Here's how the part is built. I have some questions about the finished solid (model axes, mm). A direction names the side the tool comes from. Coordinates: 2 decimals unless noted, no trailing zeros. Write each loop counter-clockwise with the first axis right and the second up, starting at its lowest first coordinate (ties: lowest second). Pieces come first, ordered by that corner, then holes.
Item 1: For faces 4 (the face through (18.255, 1.479, 74.828)), 5 (the face through (-1, 18, 98)), which set-ups out of +Z, -Z, +X, -X, +Y, -Y let a thin tool reach every point of the face, with its end or its side?
Item 2: If we mould it in two halves opening along Y, with no side actions, what happens to faces 1 (the face through (-48.4, 33, -0.5)), 2 (the face through (-1.08, 1.48, 77.46)), 3 (the face through (-1.92, 12.12, -99.01))? For each: pulls with the +Y half, pulls with the -Y half, needs draft (parallel to the pull), parting line crosses it, or undercut.
Item 3: I want a section at C-C (z = 22). Please give me the cut outline in (x, y).
Item 4: I want a section at A-A (z = -80). Please give me the cut outline in (x, y).
Item 5: Please list where these lines run through material, in increasing order: line 1 (Z direction, x = -43, y = 12.5); line 2 (X direction, y = 1, z = -26); line 3 (X direction, y = 24, z = -77).
Item 6: I want a section at B-B (x = -21). Please give me the cut outline in (y, z).
Item 7: I'm going to push flat-ended pins straight in: P1, Ø1.5, axis at x = 7, z = 65.5, coming from the -Y side; P2, Ø2, axis at x = -23, z = 25.5, coming from the +Y side. Where does each tip first touch, or does it pass through?
Item 8: I want a section at D-D (y = 25). Please give me the cut outline in (x, z), and give its area (3 significant figures).
Autodesk Inventor part; units mm, degrees
ref_plane "YZ Plane" through (0, 0, 0) normal (1, 0, 0) x (0, 1, 0)
ref_plane "XZ Plane" through (0, 0, 0) normal (0, 1, 0) x (-1, 0, 0)
ref_plane "XY Plane" through (0, 0, 0) normal (0, 0, 1) x (1, 0, 0)
sketch "스케치1" plane through (0, 0, 0) normal (0, 1, 0) x (-1, 0, 0)
  line L0 (50, 100) -> (-50, 100)
  line L1 (-50, 100) -> (-50, -100)
  line L2 (-50, -100) -> (50, -100)
  line L3 (50, -100) -> (50, 100)
  point P0 (0, 0)
  dimension "d0" = 100
  dimension "d1" = 200
extrude "돌출1" add sketch "스케치1" along normal blind 3
sketch "스케치2" plane through (0, 0, 0) normal (0, -1, 0) x (1, 0, 0)
  circle A0 centre (25, 80) radius 8.5
  circle A1 centre (35, 63) radius 1.6
  circle A2 centre (15, 63) radius 1.6
  circle A3 centre (-5, 85) radius 8.5
  circle A4 centre (4.25, 63) radius 1.6
  circle A5 centre (-14.25, 63) radius 1.6
  circle A6 centre (-35, 85) radius 8.5
  circle A7 centre (-26.25, 63) radius 1.6
  circle A8 centre (-43.75, 63) radius 1.6
  line L0 (-50, 100) -> (50, 100)
  line L1 (-50, -100) -> (-50, 100)
  line L2 (45, 30) -> (5, 30)
  line L3 (5, 30) -> (5, 10)
  line L4 (5, 10) -> (45, 10)
  line L5 (45, 10) -> (45, 30)
  circle A9 centre (2.5, 28.5) radius 1.6
  circle A10 centre (43.5, -4.5) radius 1.6
  circle A11 centre (35, 20) radius 9.6 construction
  line L6 (7, 95) -> (-17, 95) construction
  line L7 (-17, 95) -> (-17, 61) construction
  line L8 (-17, 61) -> (7, 61) construction
  line L9 (7, 61) -> (7, 95) construction
  line L10 (38.25, 96) -> (11.75, 96) construction
  line L11 (11.75, 96) -> (11.75, 60) construction
  line L12 (11.75, 60) -> (38.25, 60) construction
  line L13 (38.25, 60) -> (38.25, 96) construction
  line L14 (-23.5, 95) -> (-46.5, 95) construction
  line L15 (-46.5, 95) -> (-46.5, 61) construction
  line L16 (-46.5, 61) -> (-23.5, 61) construction
  line L17 (-23.5, 61) -> (-23.5, 95) construction
  line L18 (46.5, -24) -> (3.5, -24) construction
  line L19 (3.5, -24) -> (3.5, -96) construction
  line L20 (3.5, -96) -> (46.5, -96) construction
  line L21 (46.5, -96) -> (46.5, -24) construction
  line L22 (46.5, -24) -> (3.5, -96) construction
  line L23 (3.5, -24) -> (46.5, -96) construction
  line L24 (44.5, -29) -> (5.5, -29)
  line L25 (5.5, -29) -> (5.5, -91)
  line L26 (5.5, -91) -> (44.5, -91)
  line L27 (44.5, -91) -> (44.5, -29)
  line L28 (44.5, -29) -> (5.5, -91) construction
  line L29 (5.5, -29) -> (44.5, -91) construction
  circle A12 centre (44.4, -93.5) radius 1.5
  circle A13 centre (5.6, -93.5) radius 1.5
  circle A14 centre (5.6, -26.5) radius 1.5
  circle A15 centre (44.4, -26.5) radius 1.5
  line L30 (-29, 29.5) -> (-48, 29.5) construction
  line L31 (-48, 29.5) -> (-48, 14.5) construction
  line L32 (-48, 14.5) -> (-29, 14.5) construction
  line L33 (-29, 14.5) -> (-29, 29.5) construction
  circle A16 centre (-40, 22) radius 3
  circle A17 centre (-45.9, 16.6) radius 1.1
  circle A18 centre (-45.9, 27.4) radius 1.1
  circle A19 centre (-40, 0) radius 8.5 construction
  circle A20 centre (-40, 0) radius 3.5
  line L34 (-39, -7.5) -> (-41, -7.5)
  line L35 (-41, -7.5) -> (-41, -8.5)
  line L36 (-41, -8.5) -> (-39, -8.5)
  line L37 (-39, -8.5) -> (-39, -7.5)
  line L38 (-39, -7.5) -> (-41, -8.5) construction
  line L39 (-41, -7.5) -> (-39, -8.5) construction
  line L40 (-19, -23) -> (-40, -23)
  line L41 (-40, -23) -> (-40, -39)
  line L42 (-40, -39) -> (-19, -39)
  line L43 (-19, -39) -> (-19, -23)
  line L44 (-19, -23) -> (-40, -39) construction
  line L45 (-40, -23) -> (-19, -39) construction
  line L46 (-3, -20) -> (-45, -20) construction
  line L47 (-45, -20) -> (-45, -42) construction
  line L48 (-45, -42) -> (-3, -42) construction
  line L49 (-3, -42) -> (-3, -20) construction
  line L50 (-3, -20) -> (-45, -42) construction
  line L51 (-45, -20) -> (-3, -42) construction
  circle A21 centre (-42, -31) radius 1.5
  circle A22 centre (-13, -39) radius 1.5
  circle A23 centre (-13, -23) radius 1.5
  circle A24 centre (-15.2093, 0) radius 8.5 construction
  circle A25 centre (-15.2093, 0) radius 3.5
  line L52 (-14.2093, -7.5) -> (-16.2093, -7.5)
  line L53 (-16.2093, -7.5) -> (-16.2093, -8.5)
  line L54 (-16.2093, -8.5) -> (-14.2093, -8.5)
  line L55 (-14.2093, -8.5) -> (-14.2093, -7.5)
  line L56 (-14.2093, -7.5) -> (-16.2093, -8.5) construction
  line L57 (-16.2093, -7.5) -> (-14.2093, -8.5) construction
  point P0 (0, 0)
  point P1 (25, -60)
  point P2 (25, -60)
  point P3 (-40, -8)
  point P4 (-29.5, -31)
  point P5 (-24, -31)
  point P6 (-15.2093, -8)
  dimension "d9" = 17
  dimension "d10" = 3.2
  dimension "d11" = 3.2
  dimension "d12" = 17
  dimension "d13" = 20
  dimension "d14" = 10
  dimension "d15" = 17
  dimension "d16" = 17
  dimension "d17" = 22
  dimension "d18" = 18.5
  dimension "d19" = 9.25
  dimension "d20" = 22
  dimension "d21" = 3.2
  dimension "d22" = 3.2
  dimension "d23" = 17
  dimension "d24" = 3.2
  dimension "d25" = 22
  dimension "d26" = 3.2
  dimension "d27" = 17.5
  dimension "d28" = 8.75
  dimension "d29" = 22
  dimension "d30" = 20
  dimension "d31" = 15
  dimension "d32" = 15
  dimension "d33" = 15
  dimension "d34" = 30
  dimension "d35" = 30
  dimension "d36" = 40
  dimension "d37" = 20
  dimension "d38" = 55
  dimension "d39" = 70
  dimension "d40" = 3.2
  dimension "d41" = 3.2
  dimension "d42" = 33
  dimension "d43" = 41
  dimension "d44" = 19.2
  dimension "d45" = 10
  dimension "d46" = 10
  dimension "d47" = 24
  dimension "d48" = 34
  dimension "d49" = 12
  dimension "d50" = 10
  dimension "d51" = 26.5
  dimension "d52" = 36
  dimension "d53" = 16
  dimension "d54" = 13.25
  dimension "d55" = 23
  dimension "d56" = 34
  dimension "d57" = 11.5
  dimension "d58" = 10
  dimension "d59" = 8.5
  dimension "d60" = 32.5
  dimension "d65" = 43
  dimension "d66" = 72
  dimension "d67" = 39
  dimension "d68" = 62
  dimension "d69" = 3
  dimension "d70" = 2.1
  dimension "d71" = 2.5
  dimension "d72" = 3
  dimension "d73" = 2.5
  dimension "d74" = 2.1
  dimension "d75" = 3
  dimension "d76" = 2.5
extrude "돌출2" cut sketch "스케치2" against normal through all
sketch "스케치3" plane through (0, 3, 0) normal (0, 1, 0) x (1, 0, 0)
  line L0 (50, 100) -> (-50, 100)
  line L1 (-50, 100) -> (-50, -100)
  line L2 (50, 100) -> (-50, 100)
  line L3 (-50, 100) -> (-50, -100)
  line L4 (-50, -100) -> (50, -100)
  line L5 (50, -100) -> (50, 100)
  line L6 (48, 98) -> (-48, 98)
  line L7 (-48, 98) -> (-48, -98)
  line L8 (-48, -98) -> (48, -98)
  line L9 (48, -98) -> (48, 98)
  point P0 (0, 0)
  dimension "d139" = 2
extrude "돌출3" add sketch "스케치3" along normal blind 30
sketch "스케치4" plane through (-50, 0, 100) normal (0, 0, 1) x (1, 0, 0)
  line L0 (45, 30) -> (55, 30)
  line L1 (55, 30) -> (55, 27)
  line L2 (55, 27) -> (45, 27)
  line L3 (45, 27) -> (45, 30)
  line L4 (0, 33) -> (100, 33)
  line L5 (45, 27) -> (55, 30) construction
  line L6 (45, 30) -> (55, 27) construction
  line L7 (0, 0) -> (0, 33) construction
  point P0 (50, 0)
  point P1 (50, 28.5)
  dimension "d142" = 10
  dimension "d143" = 3
  dimension "d144" = 3
  dimension "d145" = 50
extrude "돌출4" cut sketch "스케치4" against normal through all
sketch "스케치5" plane through (50, 0, -100) normal (0, 0, -1) x (-1, 0, 0)
  line L0 (10, 23) -> (23, 23)
  line L1 (23, 23) -> (23, 10)
  line L2 (23, 10) -> (10, 10)
  line L3 (10, 10) -> (10, 23)
  line L4 (0, 0) -> (100, 0)
  line L5 (0, 0) -> (0, 33)
  circle A0 centre (53, 17) radius 5
  point P0 (50, 0)
  dimension "d148" = 13
  dimension "d149" = 13
  dimension "d150" = 10
  dimension "d151" = 10
  dimension "d152" = 10
  dimension "d153" = 17
  dimension "d154" = 25
extrude "돌출5" cut sketch "스케치5" against normal blind 30
properties part number "housing"
Answer:
1. face 4: +Y, -Y
1. face 5: +Y
2. face 1: pulls with the +Y half
2. face 2: needs draft
2. face 3: undercut
3. outline: (-50, 0) - (-43, 0) - (-43, 3) - (-48, 3) - (-48, 33) - (-50, 33) - close; (-37, 0) - (5, 0) - (5, 3) - (-37, 3) - close; (45, 0) - (50, 0) - (50, 33) - (48, 33) - (48, 3) - (45, 3) - close
4. outline: (-50, 0) - (5.5, 0) - (5.5, 3) - (-48, 3) - (-48, 33) - (-50, 33) - close; (44.5, 0) - (50, 0) - (50, 33) - (48, 33) - (48, 3) - (44.5, 3) - close
5. line 1: z = -100 to -98, 98 to 100
5. line 2: x = -50 to -40, -19 to 4.19, 7.01 to 42.99, 45.81 to 50
5. line 3: x = -50 to -48, 48 to 50
6. outline: (0, -100) - (33, -100) - (33, -98) - (3, -98) - (3, -39) - (0, -39) - close; (0, -23) - (3, -23) - (3, 98) - (33, 98) - (33, 100) - (0, 100) - close
7. P1: stops at y = 0
7. P2: stops at y = 3
8. outline: (-50, -100) - (50, -100) - (50, 100) - (-50, 100) - close; hole (-48, -98) - (48, -98) - (48, 98) - (-48, 98) - close
8. area: 1,180 mm2
